from build123d import *

# Parameters (mm, degrees)
SKETCH1_R           = 42.672
BOSS_EXTRUDE1_DEPTH = 63.5
SKETCH2_R           = 40.132
CUT_EXTRUDE1_DEPTH  = 88.601650487
SKETCH3_R           = 1.8288
SKETCH3_W           = 25.4
SKETCH3_H           = 0.762
SKETCH3_W_2         = 0.762
SKETCH3_H_2         = 45.72
CUT_EXTRUDE2_DEPTH  = 88.601650487
SKETCH4_R           = 6.35
CUT_EXTRUDE3_DEPTH  = 88.601650657
SKETCH5_R           = 6.35
CUT_EXTRUDE4_DEPTH  = 88.601650657


with BuildPart() as part:
    # Sketch1 → Boss-Extrude1 (new body)
    with BuildSketch(Plane(origin=(0, 0, 0), x_dir=(1, 0, 0), z_dir=(0, 1, 0))):
        with Locations(Location((0, 0, 0), (0, 0, 270))):
            Circle(SKETCH1_R)
    extrude(amount=BOSS_EXTRUDE1_DEPTH)

    # Sketch2 → Cut-Extrude1 (cut, through all)
    with BuildSketch(Plane(origin=(0, 0, 0), x_dir=(1, 0, 0), z_dir=(0, 1, 0))):
        with Locations(Location((0, 0, 0), (0, 0, 270))):
            Circle(SKETCH2_R)
    extrude(amount=CUT_EXTRUDE1_DEPTH, mode=Mode.SUBTRACT)

    # Sketch3 → Cut-Extrude2 (cut, through all)
    with BuildSketch(Plane.XY):
        with Locations(Location((0, 56.388, 0), (0, 0, 90.000000054))):
            Circle(SKETCH3_R)
        with Locations(Location((0, 7.112, 0), (0, 0, 90.000000054))):
            Circle(SKETCH3_R)
        with Locations((0, 52.451)):
            Rectangle(SKETCH3_W, SKETCH3_H)
        with Locations((0, 11.049)):
            Rectangle(SKETCH3_W, SKETCH3_H)
        with Locations((10.541, 31.75)):
            Rectangle(SKETCH3_W_2, SKETCH3_H_2)
        with Locations((-10.541, 31.75)):
            Rectangle(SKETCH3_W_2, SKETCH3_H_2)
    extrude(amount=CUT_EXTRUDE2_DEPTH, mode=Mode.SUBTRACT)


with BuildPart() as cut_extrude2_kept_piece:
    # of the separate pieces the step leaves, the one the design keeps (cut_extrude2_pieces_kept)
    add(part.part.solids().sort_by_distance((0, 54.5592, 42.672))[0])

    # Sketch4 → Cut-Extrude3 (cut, through all)
    with BuildSketch(Plane(origin=(0, 0, 0), x_dir=(0, -1, 0), z_dir=(-0.7071067811865488, 0, 0.7071067811865464))):
        with Locations(Location((-35.56, 0, 0), (0, 0, 270))):
            Circle(SKETCH4_R)
    extrude(amount=CUT_EXTRUDE3_DEPTH, mode=Mode.SUBTRACT)

    # Sketch5 → Cut-Extrude4 (cut, through all)
    with BuildSketch(Plane(origin=(0, 0, 0), x_dir=(0, -1, 0), z_dir=(-0.7071067811865464, 0, -0.7071067811865488))):
        with Locations(Location((-35.56, 0, 0), (0, 0, 90))):
            Circle(SKETCH5_R)
    extrude(amount=-CUT_EXTRUDE4_DEPTH, mode=Mode.SUBTRACT)


solid = cut_extrude2_kept_piece.part
Build history of the part. All positions in model axes, mm. A direction names the side the tool comes from. Give positions to 0.01 mm unless a question says otherwise; leave off trailing zeros. Order: outer loops, then holes, each group sorted by start corner. A loop starts at its lowest first (then second) coordinate and runs counter-clockwise, first axis right, second up. Notation, with made-up numbers: M 39,60 L 95,60 A25 ccw 95,76 Z; hole C -6,-20 d8. An arc over 180 degrees is marked long. Put each result on its own line as item: value.
Item 1: Cut at D-D on x = 37. Write the cut outline in (y, z).
Results are:
outline: M 0,-21.26 L 63.5,-21.26 L 63.5,-15.54 L 0,-15.54 Z; M 0,15.54 L 63.5,15.54 L 63.5,21.26 L 0,21.26 Z
Item 2: Cut at A-A on x = 0. Write the cut outline in (y, z), then the cut area to 3 significant figures.
Results are:
outline: M 0,-42.67 L 63.5,-42.67 L 63.5,-40.13 L 0,-40.13 Z; M 0,40.13 L 5.28,40.13 L 5.28,42.67 L 0,42.67 Z; M 8.94,40.13 L 10.67,40.13 L 10.67,42.67 L 8.94,42.67 Z; M 52.83,40.13 L 54.56,40.13 L 54.56,42.67 L 52.83,42.67 Z; M 58.22,40.13 L 63.5,40.13 L 63.5,42.67 L 58.22,42.67 Z
area: 197 mm2
Item 3: Drop flat-ended pins along their axis: pin 1 Ø4 at (y, z) = (35.5, -1) entering from +X; pin 2 Ø3 at (x, y) = (-5, 40) entering from -Z; pin 3 Ø0.9 at (y, z) = (54, 40) entering from -X. Give the stop position or say it passes through.
Results are:
pin 1: x = 42.67
pin 2: z = -42.53
pin 3: x = -16.02
Item 4: Cut at C-C on y = 32.5. Write the cut outline in (x, z).
Results are:
outline: M -33.85,25.98 A42.67 ccw long 33.85,25.98 L 32.04,24.17 A40.13 cw long -32.04,24.17 Z; M -25.98,33.85 L -24.17,32.04 A40.13 cw -10.92,38.62 L -10.92,41.25 A42.67 ccw Z; M 10.92,38.62 A40.13 cw 24.17,32.04 L 25.98,33.85 A42.67 ccw 10.92,41.25 Z
Item 5: Cut at B-B on z = -32. Write the cut outline in (x, y), then the cut area to 3 significant figures.
Results are:
outline: M -28.23,0 L -24.22,0 L -24.22,63.5 L -28.23,63.5 Z; M 24.22,0 L 28.23,0 L 28.23,63.5 L 24.22,63.5 Z
area: 509 mm2
Item 6: Wall check: probe 1 along X at (y, z) = (35, 0); probe 2 along X at (y, z) = (60.5, 14); probe 3 along Z at (x, y) = (19.5, 54.5). Give the ranges that are in metal, low to high.
Results are:
probe 1: -42.67 to -40.13, 40.13 to 42.67
probe 2: -40.31 to -37.61, 37.61 to 40.31
probe 3: -37.96 to -35.08, 35.08 to 37.96
Item 7: Which spindle directions (+Z, -Z, +X, -X, +Y, -Y) get a long thin tool onto all of the face, cutting with end or side? Do faces 4 (the face through (-10.922, 31, 40)), 5 (the face through (-33.233, 37.992, 24.937)). Say none if no direction does.
Results are:
face 4: +Z
face 5: none
Item 8: Pull direction Y, two halves, no side cores. Call faces 1 (the face through (0, 52.832, 41)), 2 (the face through (-28, 0, -29)), 3 (the face through (-28, 63.5, -29)): +Y half, -Y half, draft (parallel to the pull), parting line (faces both ways), or undercut.
Results are:
face 1: undercut
face 2: -Y half
face 3: +Y half
